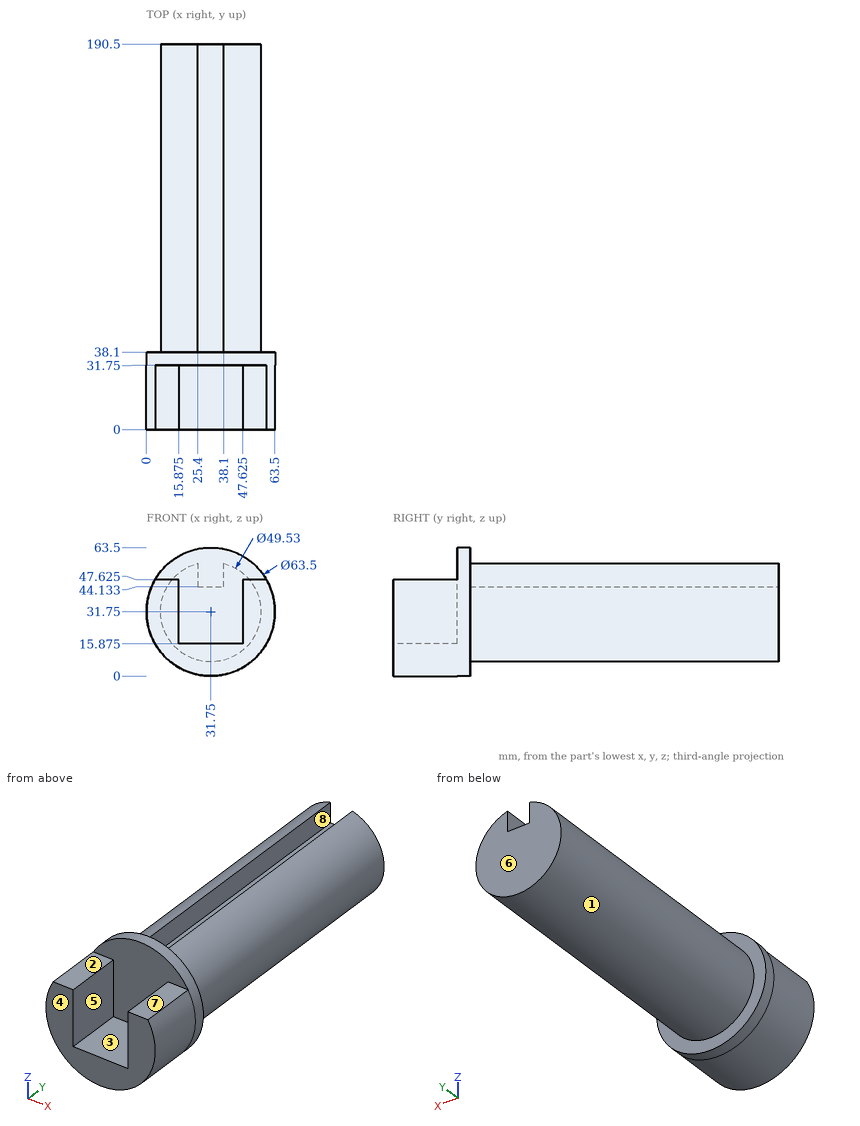
Verification items for this drawing (mm, ordinates from the low corner). A direction names the side the tool comes from. Round coordinates to 2 decimals unless told otherwise and drop trailing zeros. Write item = value, one per line. Start each with the question number.
1. Scan lines: line 1 (Y direction, x = 33.5, z = 3.5); line 2 (Y direction, x = 36.5, z = 50); line 3 (X direction, y = 153.5, z = 30.5). Record each from-to range of solid material in increasing order. Write a range as [from, to].
2. Release check for a two-part mould opening along X. For the marked faces 1, 2 and 3 record: pulls with the +X half, pulls with the -X half, needs draft (parallel to the pull), parting line crosses it, or undercut.
3. Tool access check on the marked faces 4, 5, 6, 7 and 8. Record the directions out of +Z, -Z, +X, -X, +Y, -Y that give a thin tool (end or side, any length) a straight path to the whole face; none if there is none.
4. Gauge pin test, flat ends, axial feed: pin 1 (3.5 mm diameter, centred on y = 118, z = 48, fed in from -X) (1 decimal); pin 2 (13 mm diameter, centred on x = 9, y = 23.5, fed in from +Z) (1 decimal); pin 3 (4 mm diameter, centred on x = 52, y = 121, fed in from +Z). Record the tip position at first contact, or that the pin passes through.
Results found:
q1.line_1 = [0, 38.1]
q1.line_2 = [31.75, 38.1]
q1.line_3 = [7.02, 56.48]
q2.face_1 = parting line crosses it
q2.face_2 = needs draft
q2.face_3 = undercut
q3.face_4 = +Z, -Z, +X, -X, -Y
q3.face_5 = +Z, -Y
q3.face_6 = +Z, -Z, +X, -X, +Y
q3.face_7 = +Z, +X, -X, -Y
q3.face_8 = +Z, +Y
q4.pin_1 = 11.7
q4.pin_2 = 47.6
q4.pin_3 = 48.49
